Check sheet for the modelled part. Datum: model origin and axes. Units: mm. Give positions to 0.01 mm unless a question says otherwise; leave off trailing zeros. Write each loop counter-clockwise with the first axis right and the second up, starting at its lowest first coordinate (ties: lowest second). Pieces come first, ordered by that corner, then holes. Notation, with made-up numbers: (35.5, -21.75) - (44.5, -21.75) arc R31 cw to (44.5, 9.25) - close; hole circle Ø10 at (30, 56). An arc over 180 degrees is marked (long way). Return JSON: item names as keys, results as strings. Group by question number.
```python
from build123d import *

# Parameters (mm, degrees)
SKETCH1_W           = 80
SKETCH1_H           = 40
SKETCH1_R           = 1.5
SKETCH1_R_2         = 11.5
BOSS_EXTRUDE1_DEPTH = 5


with BuildPart() as part:
    # Sketch1 → Boss-Extrude1 (new body)
    with BuildSketch(Plane.XY):
        with Locations((20, 0)):
            Rectangle(SKETCH1_W, SKETCH1_H)
        with Locations((-15.922, 15.922)):
            Circle(SKETCH1_R, mode=Mode.SUBTRACT)
        with Locations((15.922, 15.922)):
            Circle(SKETCH1_R, mode=Mode.SUBTRACT)
        with Locations((15.922, -15.922)):
            Circle(SKETCH1_R, mode=Mode.SUBTRACT)
        with Locations((-15.922, -15.922)):
            Circle(SKETCH1_R, mode=Mode.SUBTRACT)
        Circle(SKETCH1_R_2, mode=Mode.SUBTRACT)
        with BuildLine():
            Line((25, 17), (35, 17))
            ThreePointArc((35, 17), (37, 15), (35, 13))
            Line((35, 13), (25, 13))
            ThreePointArc((25, 13), (23, 15), (25, 17))
        make_face(mode=Mode.SUBTRACT)
        with BuildLine():
            Line((45, 17), (55, 17))
            ThreePointArc((55, 17), (57, 15), (55, 13))
            Line((55, 13), (45, 13))
            ThreePointArc((45, 13), (43, 15), (45, 17))
        make_face(mode=Mode.SUBTRACT)
        with BuildLine():
            Line((45, -13), (55, -13))
            ThreePointArc((55, -13), (57, -15), (55, -17))
            Line((55, -17), (45, -17))
            ThreePointArc((45, -17), (43, -15), (45, -13))
        make_face(mode=Mode.SUBTRACT)
        with BuildLine():
            Line((25, -13), (35, -13))
            ThreePointArc((35, -13), (37, -15), (35, -17))
            Line((35, -17), (25, -17))
            ThreePointArc((25, -17), (23, -15), (25, -13))
        make_face(mode=Mode.SUBTRACT)
    extrude(amount=BOSS_EXTRUDE1_DEPTH)


solid = part.part
```
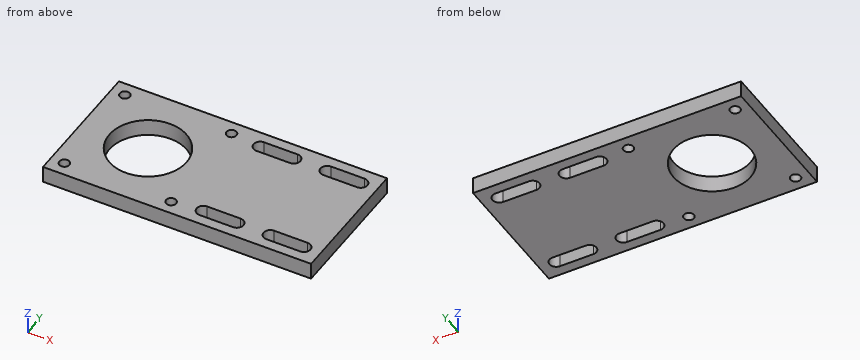
Item 1: Section check B-B on x = 50. Record the cut outline in (y, z).
Item 2: Section check D-D on y = -10. Record the cut outline in (x, z), plus the area to 3 significant figures.
Item 3: Material ranges on line 1 along Y through (x, z) = (50, 2.75); line 2 along Y through (x, z) = (0, 3.3); line 3 along X through (y, z) = (-0.5, 3.1), recorded low to high. Write a range as from..to.
Item 4: Section check C-C on z = 1.95. Count the separate pieces of the cut face and the enclosed holes in it, plus the area to 3 significant figures.
Item 5: Section check A-A on y = 0. Record the cut outline in (x, z), plus the area to 3 significant figures.
Reply:
{
 "1": {"outline": "(-20, 0) - (-17, 0) - (-17, 5) - (-20, 5) - close; (-13, 0) - (13, 0) - (13, 5) - (-13, 5) - close; (17, 0) - (20, 0) - (20, 5) - (17, 5) - close"},
 "2": {"outline": "(-20, 0) - (-5.68, 0) - (-5.68, 5) - (-20, 5) - close; (5.68, 0) - (60, 0) - (60, 5) - (5.68, 5) - close", "area": "343 mm²"},
 "3": {"line 1": "-20..-17, -13..13, 17..20", "line 2": "-20..-11.5, 11.5..20", "line 3": "-20..-11.49, 11.49..60"},
 "4": {"separate pieces": "1", "enclosed holes": "9", "area": "2,550 mm²"},
 "5": {"outline": "(-20, 0) - (-11.5, 0) - (-11.5, 5) - (-20, 5) - close; (11.5, 0) - (60, 0) - (60, 5) - (11.5, 5) - close", "area": "285 mm²"}
}
